Verification items for the finished model (mm, model axes). A direction names the side the tool comes from. Round coordinates to 2 decimals unless told otherwise and drop trailing zeros. Order: outer loops, then holes, each group sorted by start corner. A loop starts at its lowest first (then second) coordinate and runs counter-clockwise, first axis right, second up. Notation, with made-up numbers: (-4.75, 26) -> (18.25, 26) arc R15 cw to (18.25, 38) -> close; hole circle Ø6 at (-23.5, -36.5). An arc over 180 degrees is marked (long way). Return JSON: item names as keys, results as strings. Group by question number.
Item 1: Depth check by flat-ended pin: pin 1 Ø6 at (y, z) = (18.5, -79) entering from -X; pin 2 Ø3 at (y, z) = (20, -26) entering from +X. Enter the tip coordinate at first touch or a pass-through.
Item 2: Sectioned sample at A-A on y = 5.08. Record the cut outline in (x, z), plus the area to 3 significant figures.
Item 3: Draft check along Z on faces 4 (the flat face through (-50.827, 5, -104)), 5 (the cylindrical face through (-44.57, 3.15, -106.07)), 6 (the flat face through (12, 13, 18.37)). Enter one of: pulls with the +Z half, pulls with the -Z half, needs draft (parallel to the pull), parting line crosses it, or undercut.
Item 4: Access from +Z, -Z, +X, -X, +Y, -Y to the whole of each face (thin tool, end or side, straight path). Record for faces 1 (the flat face through (12, 25.4, -46)), 2 (the cylindrical face through (-44.566, 2.263, 14.755)), 3 (the cylindrical face through (69.73, 4.94, -106.72)).
Item 5: Scan line: probe 1 along X at (y, z) = (15, -66). Record every from-to range of solid material in increasing order. Write a range as from..to.
Item 6: Sectioned sample at C-C on y = 16.25. Record the cut outline in (x, z), plus the area to 3 significant figures.
Item 7: Sectioned sample at B-B on z = -54. Record the cut outline in (x, y), plus the area to 3 significant figures.
```python
from build123d import *

# Parameters (mm, degrees)
SKETCH1_W           = 101.6
SKETCH1_H           = 127
BOSS_EXTRUDE1_DEPTH = 25.4
SKETCH2_R           = 3.175
BOSS_EXTRUDE3_DEPTH = 12.7
SKETCH3_R           = 3.175
BOSS_EXTRUDE4_DEPTH = 12.7
BOSS_EXTRUDE6_START = 12.7
SKETCH4_R           = 3.175
BOSS_EXTRUDE6_DEPTH = 12.7
BOSS_EXTRUDE7_START = 12.7
SKETCH5_R           = 3.175
BOSS_EXTRUDE7_DEPTH = 12.7


with BuildPart() as part:
    # Sketch1 → Boss-Extrude1 (new body)
    with BuildSketch(Plane(origin=(0, 0, 0), x_dir=(1, 0, 0), z_dir=(0, 1, 0))):
        with Locations((12.672921109, 45.129680171)):
            Rectangle(SKETCH1_W, SKETCH1_H)
    extrude(amount=BOSS_EXTRUDE1_DEPTH)

    # Sketch2 → Boss-Extrude3 (add)
    with BuildSketch(Plane(origin=(63.472921109, 0, 0), x_dir=(0, 0, -1), z_dir=(1, 0, 0))):
        with Locations(Location((-13.290319829, 5.08, 0), (0, 0, 180))):
            Circle(SKETCH2_R)
    extrude(amount=BOSS_EXTRUDE3_DEPTH)

    # Sketch3 → Boss-Extrude4 (add)
    with BuildSketch(Plane(origin=(63.472921109, 0, 0), x_dir=(0, 0, -1), z_dir=(1, 0, 0))):
        with Locations(Location((103.549680171, 5.08, 0), (0, 0, 180))):
            Circle(SKETCH3_R)
    extrude(amount=BOSS_EXTRUDE4_DEPTH)

    # Sketch4 → Boss-Extrude6 (add)
    with BuildSketch(Plane.ZY.offset(38.127078891).offset(BOSS_EXTRUDE6_START)):
        with Locations((-103.549680171, 5.08)):
            Circle(SKETCH4_R)
    extrude(amount=-BOSS_EXTRUDE6_DEPTH)

    # Sketch5 → Boss-Extrude7 (add)
    with BuildSketch(Plane.ZY.offset(38.127078891).offset(BOSS_EXTRUDE7_START)):
        with Locations((13.290319829, 5.08)):
            Circle(SKETCH5_R)
    extrude(amount=-BOSS_EXTRUDE7_DEPTH)


solid = part.part
```
Recorded:
{
 "1": {"pin 1": "x = -38.13", "pin 2": "x = 63.47"},
 "2": {"outline": "(-50.83, -106.72) -> (-38.13, -106.72) -> (-38.13, -108.63) -> (63.47, -108.63) -> (63.47, -106.72) -> (76.17, -106.72) -> (76.17, -100.37) -> (63.47, -100.37) -> (63.47, 10.12) -> (76.17, 10.12) -> (76.17, 16.47) -> (63.47, 16.47) -> (63.47, 18.37) -> (-38.13, 18.37) -> (-38.13, 16.47) -> (-50.83, 16.47) -> (-50.83, 10.12) -> (-38.13, 10.12) -> (-38.13, -100.37) -> (-50.83, -100.37) -> close", "area": "13,200 mm²"},
 "3": {"face 4": "needs draft", "face 5": "undercut", "face 6": "pulls with the +Z half"},
 "4": {"face 1": "+Z, -Z, +X, -X, +Y", "face 2": "-X", "face 3": "+X"},
 "5": {"probe 1": "-38.13..63.47"},
 "6": {"outline": "(-38.13, -108.63) -> (63.47, -108.63) -> (63.47, 18.37) -> (-38.13, 18.37) -> close", "area": "12,900 mm²"},
 "7": {"outline": "(-38.13, 0) -> (63.47, 0) -> (63.47, 25.4) -> (-38.13, 25.4) -> close", "area": "2,580 mm²"}
}
